Can you work these out from the model? Positions are in its coordinate system, mm. Face numbers are marked on the shaded views. A direction names the side the tool comes from. Coordinates: 2 decimals unless noted, no trailing zeros. Loops run counter-clockwise (first coordinate to the right, second up) from the corner with the lowest first, then second, coordinate; pieces in that order, holes last. Notation, with made-up numbers: M 27.5,-21 L 44.5,-21 A26 ccw 44.5,-4 Z; hole C 4.5,9.25 d7. An arc over 180 degrees is marked long. Answer as a JSON object with one key per item and string values. Group by question number.
Item 1: We'd pull the mould along Z, two halves only. Please class the marked faces 1 and 2: +Z half, -Z half, draft (parallel to the pull), parting line (faces both ways), or undercut.
Item 2: Suppose I cut it at C-C (y = 71). Write out the boundary of the cut face in (x, z), then the cut area to 3 significant figures.
Item 3: If I drill on line 1 (X direction, y = -5.5, z = -0.75); line 2 (X direction, y = -0.8, z = 0); line 3 (Z direction, x = 4.75, y = 157), over which ranges is the centre line in solid material (lowest first)?
Item 4: Suppose I cut it at B-B (x = 0). Write out the boundary of the cut face in (y, z), then the cut area to 4 significant figures.
Item 5: Which directions (+Z, -Z, +X, -X, +Y, -Y) give clear straight access to the entire face, cutting with the end or side of a thin tool? Please do the marked faces 3 and 4.
Item 6: I'm going to push flat-ended pins straight in: pin 1 Ø9.5 at (x, z) = (-2, -1.5) entering from -Y; pin 2 Ø3 at (y, z) = (95, -1.5) entering from -X; pin 3 Ø10 at (x, y) = (-0.5, 171) entering from -Z. Where does each tip first touch, or does it pass through?
Item 7: Suppose I cut it at A-A (z = 0). Write out the boundary of the cut face in (x, y).
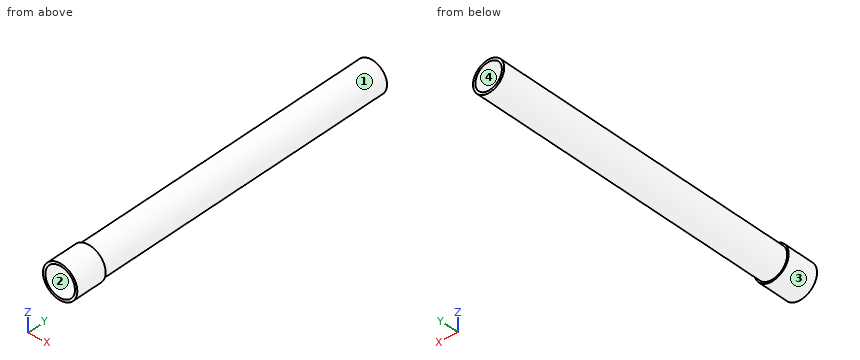
```python
from build123d import *

# Parameters (mm, degrees)
SKETCH1_R           = 10
BOSS_EXTRUDE1_DEPTH = 200
SHELL1_T            = -1.5
SKETCH2_R           = 11
BOSS_EXTRUDE2_DEPTH = 20
SHELL2_T            = -1.5


with BuildPart() as part:
    # Sketch1 → Boss-Extrude1 (new body)
    with BuildSketch(Plane(origin=(0, 0, 0), x_dir=(1, 0, 0), z_dir=(0, 1, 0))):
        with Locations(Location((0, 0, 0), (0, 0, 270))):
            Circle(SKETCH1_R)
    extrude(amount=BOSS_EXTRUDE1_DEPTH)

    # Shell1
    shell1_openings = [part.faces().sort_by_distance(p)[0] for p in [
        (0, 200, 0),
    ]]
    offset(amount=SHELL1_T, openings=shell1_openings, kind=Kind.INTERSECTION)

    # Sketch2 → Boss-Extrude2 (add)
    with BuildSketch(Plane.XZ):
        with Locations(Location((0, 0, 0), (0, 0, 270))):
            Circle(SKETCH2_R)
    extrude(amount=BOSS_EXTRUDE2_DEPTH)

    # Shell2
    shell2_openings = [part.faces().sort_by_distance(p)[0] for p in [
        (0, -20, 0),
    ]]
    offset(amount=SHELL2_T, openings=shell2_openings, kind=Kind.INTERSECTION)


solid = part.part
```
From the geometry:
{
 "1": {"face 1": "parting line", "face 2": "undercut"},
 "2": {"outline": "C 0,0 d20; hole C 0,0 d17", "area": "87.2 mm2"},
 "3": {"line 1": "-10.97 to -9.47, 9.47 to 10.97", "line 2": "-11 to -8.5, 8.5 to 11", "line 3": "-8.8 to -7.05, 7.05 to 8.8"},
 "4": {"outline": "M -20,-11 L 0,-11 L 0,-10 L 200,-10 L 200,-8.5 L 1.5,-8.5 L 1.5,8.5 L 200,8.5 L 200,10 L 0,10 L 0,11 L -20,11 L -20,9.5 L -1.5,9.5 L -1.5,8.5 L 0,8.5 L 0,-8.5 L -1.5,-8.5 L -1.5,-9.5 L -20,-9.5 Z", "area": "688.5 mm2"},
 "5": {"face 3": "+Y, -Y", "face 4": "+Y"},
 "6": {"pin 1": "y = 0", "pin 2": "x = -10", "pin 3": "z = -10"},
 "7": {"outline": "M -11,-20 L -9.5,-20 L -9.5,-1.5 L -8.5,-1.5 L -8.5,0 L 8.5,0 L 8.5,-1.5 L 9.5,-1.5 L 9.5,-20 L 11,-20 L 11,0 L 10,0 L 10,200 L 8.5,200 L 8.5,1.5 L -8.5,1.5 L -8.5,200 L -10,200 L -10,0 L -11,0 Z"}
}
